Could you check a few things on this model? Use its own coordinates, in mm. A direction names the side the tool comes from. Round coordinates to 2 decimals unless told otherwise and drop trailing zeros. Write each loop counter-clockwise with the first axis right and the second up, starting at its lowest first coordinate (ties: lowest second). Pieces come first, ordered by that corner, then holes. Notation, with made-up numbers: (61.5, 48) -> (115.5, 48) arc R27 cw to (115.5, 82) -> close; hole circle Ø6 at (19, -14). An arc over 180 degrees is marked (long way). Answer in a Markdown table with one row per item. Add a question column.
Autodesk Inventor part; units mm, degrees
ref_plane "YZ Plane" through (0, 0, 0) normal (1, 0, 0) x (0, 1, 0)
ref_plane "XZ Plane" through (0, 0, 0) normal (0, 1, 0) x (-1, 0, 0)
ref_plane "XY Plane" through (0, 0, 0) normal (0, 0, 1) x (1, 0, 0)
sketch "Sketch1" plane through (0, 0, 0) normal (0, 1, 0) x (-1, 0, 0)
  line L0 (0, 0) -> (9.5, 0)
  line L1 (9.5, 0) -> (9.5, -64)
  line L2 (9.5, -64) -> (0, -64)
  line L3 (0, -64) -> (0, 0)
  circle A0 centre (3.7, -11.5) radius 2.25
  circle A1 centre (3.7, -59.5) radius 2.25
  line L4 (3.7, -11.5) -> (3.7, -59.5) construction
  dimension "d1" = 9.5
  dimension "d2" = 64
  dimension "d3" = 4.5
  dimension "d4" = 48
  dimension "d6" = 3.7
  dimension "d17" = 4.5
extrude "Extrusion1" add sketch "Sketch1" along normal blind 12
sketch "Sketch2" plane through (-9.5, 0, 0) normal (0, 0, 1) x (1, 0, 0)
  line L0 (9.5, 12) -> (0, 12)
  line L1 (3, 12) -> (8.4, 12)
  line L2 (8.4, 12) -> (8.4, 10.8)
  line L3 (8.4, 10.8) -> (3, 10.8)
  line L4 (3, 10.8) -> (3, 12)
  line L5 (9.5, 0) -> (9.5, 12)
  line L6 (3.55, 0) -> (8.05, 0)
  line L7 (3.55, 12) -> (8.05, 12)
  line L8 (9.5, 0) -> (9.5, 12)
  line L9 (9.5, 0) -> (9.5, 12)
  line L10 (3.55, 12) -> (8.05, 12)
  line L11 (3.55, 12) -> (3.55, 0)
  line L12 (3.55, 12) -> (8.05, 12)
  line L13 (3.55, 0) -> (8.05, 0)
  line L14 (3.55, 12) -> (8.05, 12)
  line L15 (3.55, 0) -> (8.05, 0)
  line L16 (3.55, 12) -> (8.05, 12)
  line L17 (3.55, 0) -> (8.05, 0)
  dimension "d9" = 1.1
  dimension "d10" = 5.4
  dimension "d11" = 1.2
  dimension "d76" = 12
extrude "Extrusion2" cut sketch "Sketch2" against normal up to next
sketch "Sketch3" plane through (0, 0, 0) normal (0, -1, 0) x (1, 0, 0)
  circle A0 centre (-3.7, -11.5) radius 2.25
  circle A1 centre (-3.7, -11.5) radius 3.75
  circle A2 centre (-3.7, -59.5) radius 2.25
  circle A3 centre (-3.7, -59.5) radius 3.75
  point P0 (0, 0)
  dimension "d14" = 7.5
extrude "Extrusion3" cut sketch "Sketch3" against normal blind 3
fillet "Fillet1" radius 1 4 edges at (0, 1.5, -58.8897) (0, 1.5, -60.1103) (0, 1.5, -10.8897) (0, 1.5, -12.1103)
fillet "Fillet2" radius 4 2 edges at (-9.5, 6, -64) (-9.5, 6, 0)
sketch "Sketch28" plane through (0, 0, 0) normal (0, -1, 0) x (1, 0, 0)
  arc A0 (-1.5684, -56.4147) -> (0, -55.592) centre (-1, -55.592) ccw
  line L0 (0, -55.592) -> (0, -53)
  line L1 (0, -15.408) -> (0, -55.592)
  line L2 (-9.5, -60) -> (-9.5, -4)
  line L3 (0, -53) -> (-9.5, -53)
  line L4 (-9.5, -53) -> (-9.5, -34)
  line L5 (-9.5, -34) -> (0, -34)
  line L6 (0, -34) -> (0, -53)
  point P0 (0, 0)
  point P1 (0, -34)
  dimension "d107" = 2.592
  dimension "d108" = 19
extrude "Extrusion19" add sketch "Sketch28" along normal blind 20
sketch "Sketch40" plane through (0, -20, 0) normal (0, -1, 0) x (1, 0, 0)
  line L0 (0, -53) -> (-9.5, -53)
  line L1 (-9.5, -53) -> (-9.5, -73)
  line L2 (-9.5, -73) -> (0, -73)
  line L3 (0, -73) -> (0, -43)
  line L4 (0, 0) -> (0, -64)
  line L5 (0, -43) -> (-9.5, -43)
  line L6 (-9.5, -43) -> (-9.5, -53)
  line L7 (-9.5, -43) -> (0, -43)
  line L8 (0, -43) -> (0, -73)
  line L9 (0, -73) -> (-9.5, -73)
  line L10 (-9.5, -73) -> (-9.5, -43)
  dimension "d130" = 20
  dimension "d131" = 30
extrude "Extrusion21" add sketch "Sketch40" along normal blind 10
sketch "Sketch41" plane through (0, 0, -53) normal (0, 0, -1) x (-1, 0, 0)
  point P0 (0, 0)
sketch "Sketch42" plane through (0, -30, 0) normal (0, -1, 0) x (1, 0, 0)
  line L0 (-9.5, -73) -> (0, -73)
  line L1 (-9.5, -73) -> (-40.7, -73)
  line L2 (-9.5, -73) -> (21.7, -73) construction
  line L3 (-40.7, -73) -> (-40.7, -66)
  line L4 (-40.7, -66) -> (9.3, -66)
  line L5 (9.3, -66) -> (9.3, -73)
  line L6 (9.3, -73) -> (-9.5, -73)
  point P0 (0, 0)
  point P1 (0, -73)
  dimension "d134" = 31.2
  dimension "d135" = 180
  dimension "d136" = 7
  dimension "d137" = 50
  dimension "d138" = 7
extrude "Extrusion22" add sketch "Sketch42" along normal blind 7
sketch "Sketch43" plane through (-40.7, -30, -73) normal (-1, 0, 0) x (0, 0, 1)
  arc A0 (7, -7) -> (7, -57) centre (31.4949, -32) ccw
  point P0 (73, 30)
  dimension "d141" = 50
  dimension "d142" = 35
sketch "Sketch44" plane through (0, -37, 0) normal (0, -1, 0) x (1, 0, 0)
  line L0 (9.3, -73) -> (9.3, -66)
  line L1 (-40.7, -73) -> (-9.5, -73)
  line L2 (9.3, -66) -> (-40.7, -66)
  line L3 (-40.7, -66) -> (-40.7, -73)
  line L4 (-40.7, -73) -> (9.3, -73)
  line L5 (9.3, -73) -> (9.3, -66)
  point P0 (0, 0)
  point P1 (-9.5, -73)
sweep "Sweep3" add profiles "Sketch44" path "Sketch43"
sketch "Sketch54" plane through (-40.7, -30, -73) normal (-1, 0, 0) x (0, 0, 1)
  arc A0 (7, -7) -> (7, -57) centre (31.4949, -32) ccw
  line L0 (-6.4428, -57) -> (19.2704, -57)
  line L1 (19.2704, -57) -> (19.2704, -74.6848)
  line L2 (19.2704, -74.6848) -> (-6.4428, -74.6848)
  line L3 (-6.4428, -74.6848) -> (-6.4428, -57)
  point P0 (73, 30)
extrude "Extrusion25" cut sketch "Sketch54" against normal blind 104.3
chamfer "Chamfer4" distance 8.35 angle 45 1 edges at (-4.75, -20, -43)
chamfer "Chamfer5" distance 8.35 angle 45 1 edges at (-4.75, -20, -73)
properties part number "Back"
(1) Suppose I cut it at A-A, the plane x = -3.7. State how many separate pieces and enclosed holes the cut face has, then the cut area to 3 significant figures.
(2) On a 3-axis mill with a long thin cutter (end or side, diameter ignored), from which of +Z, -Z, +X, -X, +Y, -Y can I reach the whole of each face in a straight line? I mean faces 4 (the face through (-8.297, 6.084, -62.859)), 5 (the face through (-3, 6, -64)), 6 (the face through (-4, 10.8, -32)), 7 (the face through (-5, 0, -17)). Say none if no direction works.
(3) For P1, Ø6, axis at x = -4, z = -59.5, coming from the -Y side; P2, Ø1.8, axis at x = -2.5, y = -29.5, coming from the +Z side; P3, Ø4, axis at x = -22, y = -70, coming from the +Z side, each with a flat end and sliding along its axis, tell me the tip position at first contact or that it passes through.
(4) If we mould it in two halves opening along Z, with no side actions, what happens to faces 1 (the face through (-15, -34, -73)), 2 (the face through (-40.7, -57, -78)), 3 (the face through (-1, 3, -11))? For each: pulls with the +Z half, pulls with the -Z half, needs draft (parallel to the pull), parting line crosses it, or undercut.
(5) Suppose I cut it at D-D, the plane x = 2. Please give me the cut outline in (y, z).
(6) I need wall thicknesses on L1, parallel to Z at x = -3.7, y = 0.9; L2, parallel to X at y = -2, z = -49; L3, parallel to X at y = 5.75, z = -59.5. Which ranges of each line are inside material? Lowest first, please.
(7) Suppose I cut it at C-C, the plane z = -28. Please give me the cut outline in (x, y), then the cut area to 3 significant figures.
(8) Suppose I cut it at B-B, the plane z = -11.5. Please give me the cut outline in (x, y).
Response:
| question | item | result |
|---|---|---|
| 1 | separate pieces | 3 |
| 1 | enclosed holes | 0 |
| 1 | area | 1,590 mm² |
| 2 | face 4 | -Z, -X, +Y |
| 2 | face 5 | -Z, +X, -X, +Y |
| 2 | face 6 | +Z, -Z, +Y |
| 2 | face 7 | +Z, +X, -X, -Y |
| 3 | P1 | y = -30 |
| 3 | P2 | z = -43 |
| 3 | P3 | z = -75.05 |
| 4 | face 1 | pulls with the -Z half |
| 4 | face 2 | needs draft |
| 4 | face 3 | undercut |
| 5 | outline | (-87, -73) arc R40.21 ccw to (-37, -73) -> (-30, -73) -> (-30, -66) -> (-37, -66) arc R35 cw to (-87, -66) -> close |
| 6 | L1 | -64 to -63.25, -55.75 to -15.25, -7.75 to 0 |
| 6 | L2 | -9.5 to 0 |
| 6 | L3 | -9.5 to -5.95, -1.45 to 0 |
| 7 | outline | (-9.5, 0) -> (0, 0) -> (0, 12) -> (-1.1, 12) -> (-1.1, 10.8) -> (-6.5, 10.8) -> (-6.5, 12) -> (-9.5, 12) -> close |
| 7 | area | 108 mm² |
| 8 | outline | (-9.5, 0) -> (-7.45, 0) -> (-7.45, 3) -> (-5.95, 3) -> (-5.95, 10.8) -> (-6.5, 10.8) -> (-6.5, 12) -> (-9.5, 12) -> close; (-1.45, 3) -> (0, 3) -> (0, 12) -> (-1.1, 12) -> (-1.1, 10.8) -> (-1.45, 10.8) -> close |
